Geometry check sheet. Reference: the model listing, model coordinates, mm. A direction names the side the tool comes from. Round coordinates to 2 decimals unless told otherwise and drop trailing zeros. Loops run counter-clockwise (first coordinate to the right, second up) from the corner with the lowest first, then second, coordinate; pieces in that order, holes last. Notation, with made-up numbers: M 26.25,54 L 31.25,54 A30 ccw 31.25,83 Z; hole C 13.5,57.5 d11. An arc over 180 degrees is marked long. Use one line per item in the form item = value. Start each with the question number.
1. Cross-section at B-B (y = 0). Record the boundary of the cut face in (x, z) (1 decimal), then the cut area to 3 significant figures.
2. Cross-section at A-A (x = 1.3). Record the boundary of the cut face in (y, z) (3 decimals).
3. Material ranges on line 1 (Y direction, x = 1.15, z = 0); line 2 (Z direction, x = 1.3, y = 3.5); line 3 (Z direction, x = 1.55, y = -7.5), recorded low to high.
4. Draft check along Z on faces 4 (the flat face through (0.78, -14.66, -37.42)), 5 (the flat face through (1.588, 0, -28)), 6 (the flat face through (0.78, -19.67, -56.7)). Enter one of: pulls with the +Z half, pulls with the -Z half, needs draft (parallel to the pull), parting line crosses it, or undercut.
5. Cross-section at C-C (z = 0). Record the boundary of the cut face in (x, y), then the cut area to 3 significant figures.
6. Go/stop test with a flat-tipped pin: pin 1 (10 mm diameter, centred on y = 11.5, z = -45.5, fed in from +X). Record where the tip stops, or that it passes through.
7. Cross-section at D-D (z = -59.5). Record the boundary of the cut face in (x, y), then the cut area to 3 significant figures.
8. Set-up check for faces 1 (the flat face through (0.78, 14.19, -40.11)), 2 (the flat face through (0.783, -17.106, -46.793)), 3 (the flat face through (0.78, -13.82, -28.03)): record each of +Z, -Z, +X, -X, +Y, -Y from which the full face is reachable in a straight line by a thin tool's end or side.
```python
from build123d import *

# Parameters (mm, degrees)
BOSS_EXTRUDE1_DEPTH  = 1.5875
M8_CLEARANCE_HOLE1_D = 8.4


with BuildPart() as part:
    # Sketch1 → Boss-Extrude1 (new body)
    with BuildSketch(Plane(origin=(0, 0, 0), x_dir=(0, 0, -1), z_dir=(1, 0, 0))):
        with BuildLine():
            ThreePointArc((-7.638168997, 5.690694103), (-8.852669963, -3.515090259), (-1.653998892, -9.380293847))
            Line((-1.653998892, -9.380293847), (27.892706706, -14.590175236))
            Line((27.892706706, -14.590175236), (28.168373188, -13.026792928))
            Line((28.168373188, -13.026792928), (46.928960883, -16.334790712))
            Line((46.928960883, -16.334790712), (46.653294401, -17.89817302))
            Line((46.653294401, -17.89817302), (67.035446451, -21.492096351))
            ThreePointArc((67.035446451, -21.492096351), (63.524537099, -13.489075558), (66.01577467, -5.112407863))
            Line((66.01577467, -5.112407863), (13.47644349, 34.0311699))
            Line((13.47644349, 34.0311699), (-7.638168997, 5.690694103))
        make_face()
    extrude(amount=BOSS_EXTRUDE1_DEPTH)

    # M8 Clearance Hole1 (through all)
    with Locations(Plane(origin=(1.5875, 0, 0), x_dir=(0, 0, -1), z_dir=(1, 0, 0))):
        with Locations((0, 0)):
            Hole(M8_CLEARANCE_HOLE1_D / 2)


solid = part.part
```
Reported:
q1.outline = M 0,-59.2 L 1.6,-59.2 L 1.6,-4.2 L 0,-4.2 Z; M 0,4.2 L 1.6,4.2 L 1.6,9.5 L 0,9.5 Z
q1.area = 95.7 mm²
q2.outline = M -21.492,-67.035 A12.7 cw -5.112,-66.016 L 34.031,-13.476 L 5.691,7.638 A9.525 ccw -9.38,1.654 L -14.59,-27.893 L -13.027,-28.168 L -16.335,-46.929 L -17.898,-46.653 Z; hole C 0,0 d8.4
q3.line_1 = -9.67 to -4.2, 4.2 to 15.94
q3.line_2 = -54.46 to -2.32, 2.32 to 8.86
q3.line_3 = -64.61 to 5.87
q4.face_4 = undercut
q4.face_5 = needs draft
q4.face_6 = pulls with the +Z half
q5.outline = M 0,-9.67 L 1.59,-9.67 L 1.59,-4.2 L 0,-4.2 Z; M 0,4.2 L 1.59,4.2 L 1.59,15.94 L 0,15.94 Z
q5.area = 27.3 mm²
q6.pin_1 = 1.59
q7.outline = M 0,-20.16 L 1.59,-20.16 L 1.59,-0.26 L 0,-0.26 Z
q7.area = 31.6 mm²
q8.face_1 = -Z, +X, -X, +Y
q8.face_2 = +Z, +X, -X
q8.face_3 = +X, -X, -Y
